Geometry: final body of the model. Coordinates: model frame, mm. Face numbers are marked on the shaded views. Coordinates: 2 decimals unless noted, no trailing zeros. Write item = value, one per line. Start each with the question number.
Item 1: Ray query, L1, parallel to Z at x = 9.5, y = 2; L2, parallel to Y at x = 0, z = 36.5; L3, parallel to Y at x = 0, z = 36.2. Return the intervals inside material, ascending. Write a range as [from, to].
Item 2: First-contact query: pin 1 Ø12.5 at (x, y) = (-7.5, -7) entering from +Z. Flat tip, straight axial feed; report the tip coordinate or a pass-through.
Item 3: Pull-direction query (Y, two-part tool) for the marked faces 1, 2, 3 and 4; classes: +Y half, -Y half, draft (parallel to the pull), parting line (faces both ways), or undercut.
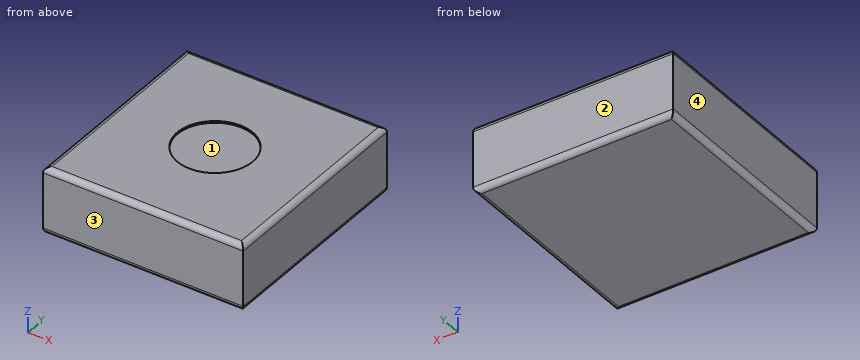
from build123d import *

# Parameters (mm, degrees)
SKETCH_1_W          = 112
SKETCH_1_H          = 117
EXTRUDE_1_DEPTH     = 37
FILLET_1_R          = 3
FILLET_2_R          = 3
SKETCH_2_R          = 21.074583211
CUT_EXTRUDE_1_DEPTH = 1


with BuildPart() as part:
    # 草图1 → 凸台-拉伸1 (new body)
    with BuildSketch(Plane.XY):
        Rectangle(SKETCH_1_W, SKETCH_1_H)
    extrude(amount=EXTRUDE_1_DEPTH)

    # 圆角1
    fillet_1_edges = [part.edges().sort_by_distance(p)[0] for p in [
        (-56, 0, 37),
        (0, -58.5, 37),
        (56, 0, 37),
        (0, 58.5, 37),
    ]]
    fillet(fillet_1_edges, radius=FILLET_1_R)

    # 圆角2
    fillet_2_edges = [part.edges().sort_by_distance(p)[0] for p in [
        (0, -58.5, 0),
        (-56, 0, 0),
        (0, 58.5, 0),
        (56, 0, 0),
    ]]
    fillet(fillet_2_edges, radius=FILLET_2_R)

    # 草图2 → 切除-拉伸1 (cut)
    with BuildSketch(Plane.XY.offset(37)):
        Circle(SKETCH_2_R)
    extrude(amount=-CUT_EXTRUDE_1_DEPTH, mode=Mode.SUBTRACT)


solid = part.part
Responses:
q1.L1 = [0, 36]
q1.L2 = [-57.16, -21.07], [21.07, 57.16]
q1.L3 = [-57.54, -21.07], [21.07, 57.54]
q2.pin_1 = 36
q3.face_1 = undercut
q3.face_2 = +Y half
q3.face_3 = -Y half
q3.face_4 = draft
